Can you work these out from the model? Positions are in its coordinate system, mm. A direction names the side the tool comes from. Round coordinates to 2 decimals unless told otherwise and drop trailing zeros. Order: outer loops, then holes, each group sorted by start corner. A loop starts at its lowest first (then second) coordinate and runs counter-clockwise, first axis right, second up.
from build123d import *
from build123d.topology import SkipClean

# Parameters (mm, degrees)
SKETCH1_R           = 125
SKETCH1_R_2         = 20
BOSS_EXTRUDE1_DEPTH = 4
SKETCH2_W           = 8
SKETCH2_H           = 40
BOSS_EXTRUDE2_DEPTH = 99
SKETCH3_R           = 11
CUT_EXTRUDE1_DEPTH  = 287.646559372
BOSS_EXTRUDE3_START = 22
BOSS_EXTRUDE3_DEPTH = 4
BOSS_EXTRUDE4_START = -22
SKETCH5_3_R         = 11
BOSS_EXTRUDE4_DEPTH = 4


with BuildPart() as part:
    # Sketch1 → Boss-Extrude1 (new, symmetric)
    with BuildSketch(Plane(origin=(0, 0, 0), x_dir=(1, 0, 0), z_dir=(0, 1, 0))):
        with Locations(Location((0, 0, 0), (0, 0, 270))):
            Circle(SKETCH1_R)
        with Locations(Location((0, 0, 0), (0, 0, 270))):
            Circle(SKETCH1_R_2, mode=Mode.SUBTRACT)
    extrude(amount=BOSS_EXTRUDE1_DEPTH, both=True)

    # Sketch2 → Boss-Extrude2 (add)
    with BuildSketch(Plane.XZ.offset(4)):
        with Locations((107.5, 0)):
            Rectangle(SKETCH2_W, SKETCH2_H)
        with Locations((-107.5, 0)):
            Rectangle(SKETCH2_W, SKETCH2_H)
    extrude(amount=BOSS_EXTRUDE2_DEPTH)

    # Sketch3 → Cut-Extrude1 (cut, through all)
    with BuildSketch(Plane(origin=(111.5, 0, 0), x_dir=(0, 0, -1), z_dir=(1, 0, 0))):
        with Locations((0, -83)):
            Circle(SKETCH3_R)
        with BuildLine():
            Line((20, -103), (20, -83))
            ThreePointArc((20, -83), (14.142135624, -97.142135624), (0, -103))
            Line((0, -103), (20, -103))
        make_face()
        with BuildLine():
            ThreePointArc((0, -103), (-14.142135624, -97.142135624), (-20, -83))
            Line((-20, -83), (-20, -103))
            Line((-20, -103), (0, -103))
        make_face()
    extrude(amount=-CUT_EXTRUDE1_DEPTH, mode=Mode.SUBTRACT)

    # Sketch5 → Boss-Extrude3 (add, symmetric)
    with SkipClean():  # the faces are left unmerged after this step: merging them gives an invalid solid
        with BuildSketch(Plane(origin=(0, 0, 0), x_dir=(0, 0, -1), z_dir=(1, 0, 0)).offset(BOSS_EXTRUDE3_START)):
            with BuildLine():
                Line((-97, -4), (-118.540084836, -4))
                ThreePointArc((-118.540084836, -4), (-139.773172479, -114.051826294), (-124.070028997, -225.02776858))
                ThreePointArc((-124.070028997, -225.02776858), (-120.91053372, -206.881628956), (-104.256328594, -199.013830961))
                Line((-104.256328594, -199.013830961), (-97, -4))
            make_face()
            with BuildLine():
                Line((-75.459915164, -4), (-97, -4))
                Line((-97, -4), (-104.256328594, -199.013830961))
                ThreePointArc((-104.256328594, -199.013830961), (-92.881628956, -203.08946628), (-85.929971003, -212.97223142))
                ThreePointArc((-85.929971003, -212.97223142), (-99.503702638, -107.543747619), (-75.459915164, -4))
            make_face()
            with BuildLine():
                ThreePointArc((-104.256328594, -199.013830961), (-120.91053372, -206.881628956), (-124.070028997, -225.02776858))
                Line((-124.070028997, -225.02776858), (-115.488515948, -222.315272719))
                ThreePointArc((-115.488515948, -222.315272719), (-113.750793546, -212.334895926), (-104.590980727, -208.007607029))
                Line((-104.590980727, -208.007607029), (-104.256328594, -199.013830961))
            make_face()
            with BuildLine():
                ThreePointArc((-85.929971003, -212.97223142), (-92.881628956, -203.08946628), (-104.256328594, -199.013830961))
                Line((-104.256328594, -199.013830961), (-104.590980727, -208.007607029))
                ThreePointArc((-104.590980727, -208.007607029), (-98.334895926, -210.249206454), (-94.511484052, -215.684727281))
                Line((-94.511484052, -215.684727281), (-85.929971003, -212.97223142))
            make_face()
            with BuildLine():
                Line((-115.488515948, -222.315272719), (-124.070028997, -225.02776858))
                ThreePointArc((-124.070028997, -225.02776858), (-101.950457406, -238.766139987), (-85, -219))
                ThreePointArc((-85, -219), (-85.233860013, -215.950457406), (-85.929971003, -212.97223142))
                Line((-85.929971003, -212.97223142), (-94.511484052, -215.684727281))
                ThreePointArc((-94.511484052, -215.684727281), (-94.128623007, -217.322751573), (-94, -219))
                ThreePointArc((-94, -219), (-103.322751573, -229.871376993), (-115.488515948, -222.315272719))
            make_face()
        extrude(amount=BOSS_EXTRUDE3_DEPTH, both=True)

    # Sketch5_3 → Boss-Extrude4 (add, symmetric)
    with BuildSketch(Plane(origin=(0, 0, 0), x_dir=(0, 0, -1), z_dir=(1, 0, 0)).offset(BOSS_EXTRUDE4_START)):
        with BuildLine():
            ThreePointArc((-124.070028997, -225.02776858), (-98.97223142, -238.070028997), (-85.929971003, -212.97223142))
            ThreePointArc((-85.929971003, -212.97223142), (-99.503702638, -107.543747619), (-75.459915164, -4))
            Line((-75.459915164, -4), (-118.540084836, -4))
            ThreePointArc((-118.540084836, -4), (-139.773172479, -114.051826294), (-124.070028997, -225.02776858))
        make_face()
        with Locations((-105, -219)):
            Circle(SKETCH5_3_R, mode=Mode.SUBTRACT)
    extrude(amount=BOSS_EXTRUDE4_DEPTH, both=True)


solid = part.part
(1) I want a section at D-D, the plane y = -64. List the corners of the cut face in (x, z) for me.
(2) If we mould it in two halves opening along X, with no side actions, what happens to faces 5 (the face through (-21.944, -109.038, 99.575)), 6 (the face through (5.5, 0.06, -124.88)), 7 (the face through (-103.5, -53, 0))? For each: pulls with the +X half, pulls with the -X half, needs draft (parallel to the pull), parting line crosses it, or undercut.
(3) I want a section at B-B, the plane z = -7. List the corners of the cut face in (x, y) for me (3 decimals), plus the area to 3 significant figures.
(4) I want a section at A-A, the plane x = 0. List the corners of the cut face in (y, z) for me, plus the area to 3 significant figures.
(5) I want a section at C-C, the plane y = -110. List the corners of the cut face in (x, z) for me.
(6) I'm going to push flat-ended pins straight in: pin 1 Ø1 at (x, z) = (14, 98.5) entering from -Y; pin 2 Ø4 at (x, y) = (109, -37.5) entering from +Z; pin 3 Ø2.5 at (x, y) = (107, -34) entering from -Z. Where does each tip first touch, or does it pass through?
(7) Please list where these lines run through material, in increasing order: probe 1 along Y at (x, z) = (-20, 105); probe 2 along Y at (x, z) = (-108, 0); probe 3 along X at (y, z) = (-52.5, 123).
(8) On a 3-axis mill with a long thin cutter (end or side, diameter ignored), from which of +Z, -Z, +X, -X, +Y, -Y can I reach the whole of each face in a straight line? I mean faces 1 (the face through (-26, -120, 115)), 2 (the face through (103.5, -53, 0)), 3 (the face through (-108, -43, -20)), 4 (the face through (107, -43, 20)). Say none if no direction works.
Ans:
1. outline: (-111.5, -20) - (-103.5, -20) - (-103.5, 20) - (-111.5, 20) - close; (-26, 94.11) - (-18, 94.11) - (-18, 134.8) - (-26, 134.8) - close; (18, 94.11) - (26, 94.11) - (26, 134.8) - (18, 134.8) - close; (103.5, -20) - (111.5, -20) - (111.5, 20) - (103.5, 20) - close
2. face 5: needs draft
2. face 6: parting line crosses it
2. face 7: undercut
3. outline: (-124.804, -4) - (-111.5, -4) - (-111.5, -74.515) - (-103.5, -74.515) - (-103.5, -4) - (-18.735, -4) - (-18.735, 4) - (-124.804, 4) - close; (-111.5, -101.735) - (-103.5, -101.735) - (-103.5, -91.485) - (-111.5, -91.485) - close; (18.735, -4) - (103.5, -4) - (103.5, -74.515) - (111.5, -74.515) - (111.5, -4) - (124.804, -4) - (124.804, 4) - (18.735, 4) - close; (103.5, -101.735) - (111.5, -101.735) - (111.5, -91.485) - (103.5, -91.485) - close
3. area: 2,990 mm2
4. outline: (-4, -125) - (4, -125) - (4, -20) - (-4, -20) - close; (-4, 20) - (4, 20) - (4, 125) - (-4, 125) - close
4. area: 1,680 mm2
5. outline: (-26, 99.62) - (-18, 99.62) - (-18, 139.65) - (-26, 139.65) - close; (18, 99.62) - (26, 99.62) - (26, 139.65) - (18, 139.65) - close
6. pin 1: stops at y = -4
6. pin 2: stops at z = 20
6. pin 3: stops at z = -20
7. probe 1: y = -239 to -230, -208 to 4
7. probe 2: y = -103 to -94, -72 to 4
7. probe 3: x = -26 to -18, 18 to 26
8. face 1: +Z, -Z, -X, -Y
8. face 2: +Z, -Z, -Y
8. face 3: -Z, +X, -X, -Y
8. face 4: +Z, +X, -X, -Y
